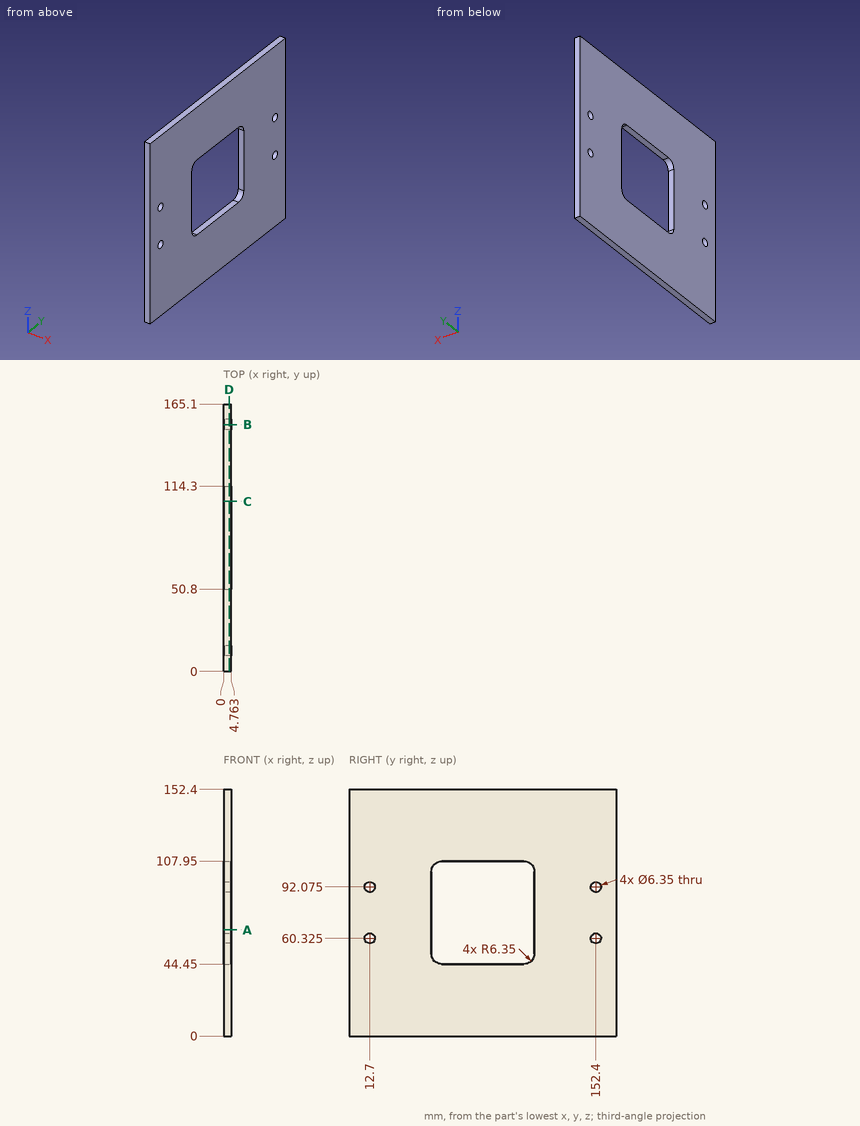
The figure shows three views and two pictorial views of one solid part (mm, origin at its lowest corner). Answer the questions. Give positions to 0.01 mm unless a question says otherwise; leave off trailing zeros. Order: outer loops, then holes, each group sorted by start corner. A loop starts at its lowest first (then second) coordinate and runs counter-clockwise, first axis right, second up. Notation, with made-up numbers: (69.25, -33.75) -> (96.25, -33.75) arc R29 cw to (96.25, 4.25) -> close; hole circle Ø11 at (13.25, 33). An arc over 180 degrees is marked (long way). Answer as CSV lines item,"result". Start each with the question number.
(1) Section C-C, the plane y = 105 is taken. Write down the section's boundary in (x, z).
(2) Section A-A, the plane z = 65.5 is taken. Write down the section's boundary in (x, y).
(3) Section B-B, the plane y = 152.4 is taken. Write down the section's boundary in (x, z).
(4) Section D-D, the plane x = 3.4 is taken. Give the number of separate pieces and of enclosed holes in the cut face, plus the area to 3 significant figures.
(5) Consider line 1 along Z through (x, y) = (1.65, 152.4); line 2 along Y through (x, z) = (4.45, 66.5); line 3 along Z through (x, y) = (3.4, 92). Determine where each line is inside the solid, lowest interval first.
Entries:
1,outline,"(0, 0) -> (4.76, 0) -> (4.76, 44.45) -> (0, 44.45) -> close; (0, 107.95) -> (4.76, 107.95) -> (4.76, 152.4) -> (0, 152.4) -> close"
2,outline,"(0, 0) -> (4.76, 0) -> (4.76, 50.8) -> (0, 50.8) -> close; (0, 114.3) -> (4.76, 114.3) -> (4.76, 165.1) -> (0, 165.1) -> close"
3,outline,"(0, 0) -> (4.76, 0) -> (4.76, 57.15) -> (0, 57.15) -> close; (0, 63.5) -> (4.76, 63.5) -> (4.76, 88.9) -> (0, 88.9) -> close; (0, 95.25) -> (4.76, 95.25) -> (4.76, 152.4) -> (0, 152.4) -> close"
4,separate pieces,"1"
4,enclosed holes,"5"
4,area,"21,000 mm²"
5,line 1,"0 to 57.15, 63.5 to 88.9, 95.25 to 152.4"
5,line 2,"0 to 50.8, 114.3 to 165.1"
5,line 3,"0 to 44.45, 107.95 to 152.4"
